from build123d import *

# Parameters (mm, degrees)
CROQUIS1_W                 = 15
CROQUIS1_H                 = 92
CROQUIS1_W_2               = 13
CROQUIS1_H_2               = 90
EXTRUIR_L_MINA1_DEPTH      = 10
CROQUIS2_W                 = 9
CROQUIS2_H                 = 13
CORTAR_EXTRUIR2_DEPTH      = 94.594871654
CROQUIS5_W                 = 13
CROQUIS5_H                 = 90
SALIENTE_EXTRUIR1_DEPTH    = 1
CORTAR_EXTRUIR3_DEPTH      = 93.509458976
CORTAR_EXTRUIR3_DEPTH_BACK = 93.509458976
CROQUIS6_R                 = 2.75


with BuildPart() as part:
    # Croquis1 → Extruir-Lámina1 (new body)
    with BuildSketch(Plane.YZ):
        with Locations((6.5, 45)):
            Rectangle(CROQUIS1_W, CROQUIS1_H)
        with Locations((6.5, 45)):
            Rectangle(CROQUIS1_W_2, CROQUIS1_H_2, mode=Mode.SUBTRACT)
    extrude(amount=EXTRUIR_L_MINA1_DEPTH)

    # Croquis2 → Cortar-Extruir2 (cut, through all)
    with BuildSketch(Plane(origin=(0, 0, -1), x_dir=(1, 0, 0), z_dir=(0, 0, -1))):
        with Locations((5.5, -6.5)):
            Rectangle(CROQUIS2_W, CROQUIS2_H)
    extrude(amount=-CORTAR_EXTRUIR2_DEPTH, mode=Mode.SUBTRACT)

    # Croquis5 → Saliente-Extruir1 (add)
    with BuildSketch(Plane(origin=(0, 0, 0), x_dir=(0, -1, 0), z_dir=(-1, 0, 0))):
        with Locations((-6.5, 45)):
            Rectangle(CROQUIS5_W, CROQUIS5_H)
    extrude(amount=-SALIENTE_EXTRUIR1_DEPTH)

    # Croquis6 → Cortar-Extruir3 (cut, two sides: drawn at the far end of the back side and taken through both)
    with BuildSketch(Plane.YZ.offset(1).offset(-CORTAR_EXTRUIR3_DEPTH_BACK)):
        with Locations((6.5, 17)):
            Circle(CROQUIS6_R)
        with Locations((6.5, 81)):
            Circle(CROQUIS6_R)
        with Locations((6.5, 6)):
            Circle(CROQUIS6_R)
    extrude(amount=CORTAR_EXTRUIR3_DEPTH + CORTAR_EXTRUIR3_DEPTH_BACK, mode=Mode.SUBTRACT)


solid = part.part
Check sheet for the modelled part. Datum: model origin and axes. Units: mm. A direction names the side the tool comes from. Give positions to 0.01 mm unless a question says otherwise; leave off trailing zeros. Loops run counter-clockwise (first coordinate to the right, second up) from the corner with the lowest first, then second, coordinate; pieces in that order, holes last. Notation, with made-up numbers: M 43.5,86.5 L 48.5,86.5 A29 ccw 48.5,119.5 Z; hole C 73.5,69 d9. An arc over 180 degrees is marked long. Answer as a JSON object with one key per item and string values. Group by question number.
Q1. Cross-section at A-A on x = 7. Record the cut outline in (y, z).
Q2. Cross-section at C-C on y = 6.5. Record the cut outline in (x, z), then the cut area to 3 significant figures.
Q3. Go/stop test with flat-tipped pins: P1, Ø7, axis at y = 6.5, z = 6, coming from the +X side; P2, Ø5, axis at y = 6.5, z = 81, coming from the +X side. Record where each tip stops, or that it passes through.
Q4. Access from +Z, -Z, +X, -X, +Y, -Y to the whole of each face (thin tool, end or side, straight path). Record for faces 5 (the flat face through (5, 0, 44)), 6 (the flat face through (0.5, 6.5, -1)).
Q5. Cross-section at D-D on y = 3. Record the cut outline in (x, z).
Q6. Material ranges on line 1 along Z through (x, y) = (0.6, 6.5); line 2 along Y through (x, z) = (0.6, 6); line 3 along Y through (x, z) = (8, 18.5), recorded low to high. Write a range as [from, to].
Q7. Release check for a two-part mould opening along Y. For faces 1 (the cylindrical face through (0.49, 9.12, 81.83)), 2 (the flat face through (5, -1, 44)), 3 (the flat face through (0.5, 6.5, 91)), 4 (the flat face through (5, 14, 44)) record: released by +Y, released by -Y, zero draft, split by the parting line, or undercut.
Q8. Cross-section at B-B on z = 17. Record the cut outline in (x, y), then the cut area to 3 significant figures.
Evaluation:
{
 "1": {"outline": "M -1,-1 L 0,-1 L 0,91 L -1,91 Z; M 13,-1 L 14,-1 L 14,91 L 13,91 Z"},
 "2": {"outline": "M 0,-1 L 1,-1 L 1,3.25 L 0,3.25 Z; M 0,8.75 L 1,8.75 L 1,14.25 L 0,14.25 Z; M 0,19.75 L 1,19.75 L 1,78.25 L 0,78.25 Z; M 0,83.75 L 1,83.75 L 1,91 L 0,91 Z", "area": "75.5 mm2"},
 "3": {"P1": "stops at x = 1", "P2": "passes through"},
 "4": {"face 5": "+Z, -Z, +X", "face 6": "-Z, +X, -X, +Y, -Y"},
 "5": {"outline": "M 0,-1 L 1,-1 L 1,91 L 0,91 Z"},
 "6": {"line 1": "z = [-1, 3.25], [8.75, 14.25], [19.75, 78.25], [83.75, 91]", "line 2": "y = [-1, 3.75], [9.25, 14]", "line 3": "y = [-1, 0], [13, 14]"},
 "7": {"face 1": "undercut", "face 2": "released by -Y", "face 3": "zero draft", "face 4": "released by +Y"},
 "8": {"outline": "M 0,-1 L 10,-1 L 10,0 L 1,0 L 1,3.75 L 0,3.75 Z; M 0,9.25 L 1,9.25 L 1,13 L 10,13 L 10,14 L 0,14 Z", "area": "27.5 mm2"}
}
